Work out the finished part from the listing and answer in its coordinate system (mm). Face numbers are marked on the shaded views. A direction names the side the tool comes from. Give positions to 0.01 mm unless a question says otherwise; leave off trailing zeros. Loops run counter-clockwise (first coordinate to the right, second up) from the corner with the lowest first, then second, coordinate; pieces in that order, holes last. Notation, with made-up numbers: M -33.5,-7 L -8.5,-7 A22 ccw -8.5,28 Z; hole C 18.5,-1 d6. An arc over 180 degrees is marked long. Write item = value, one per line. Start each with the question number.
1. Flat-ended cylindrical pins translate along their axes: pin 1 Ø2 at (x, z) = (1.5, 4) entering from -Y; pin 2 Ø4.5 at (x, z) = (-14.5, 2.5) entering from +Y; pin 3 Ø3 at (y, z) = (5, 1.5) entering from +X. Find the tip coordinate at first contact, or state that the pin passes through.
2. The mould has two halves that part along X. Classify the marked faces 4, 5 and 6: released by +X, released by -X, zero draft, split by the parting line, or undercut.
3. Section B-B on z = 6.75 is taken. Determine the outline of the cut face in (x, y), plus the area to 3 significant figures.
4. Section D-D on z = 4.5 is taken. Determine the outline of the cut face in (x, y).
5. Consider L1, parallel to Y at x = 4.5, z = 7.5; L2, parallel to Z at x = -14, y = -4.7; L3, parallel to X at y = 2.5, z = 2.75. Determine where each line is inside the solid, lowest interval first. Write a range as [from, to].
6. For the marked faces 1, 2 and 3, determine the directions among +Z, -Z, +X, -X, +Y, -Y from which every point of the face is accessible in a straight line to the end or side of a thin tool.
7. Section C-C on y = -1.35 is taken. Determine the outline of the cut face in (x, z).
8. Section A-A on x = 0 is taken. Determine the outline of the cut face in (y, z), plus the area to 3 significant figures.
```python
from build123d import *

# Parameters (mm, degrees)
SKETCH3_W                                            = 18
SKETCH3_H                                            = 13
BOSS_EXTRUDE1_DEPTH                                  = 9
SKETCH9_W                                            = 12.6
SKETCH9_H                                            = 10.3
CUT_EXTRUDE2_DEPTH                                   = 6
SKETCH10_R                                           = 2.25
CUT_EXTRUDE3_DEPTH                                   = 13.619429464
CSK_FOR_M1_6_COUNTERSUNK_FLAT_HEAD_SCREW_D           = 2
CSK_FOR_M1_6_COUNTERSUNK_FLAT_HEAD_SCREW_CSINK_D     = 3.6
CSK_FOR_M1_6_COUNTERSUNK_FLAT_HEAD_SCREW_CSINK_ANGLE = 90
SKETCH14_W                                           = 9
SKETCH14_H                                           = 4
BOSS_EXTRUDE2_DEPTH                                  = 10
M1_6_CLEARANCE_HOLE1_D                               = 2


with BuildPart() as part:
    # Sketch3 → Boss-Extrude1 (new body)
    with BuildSketch(Plane.XY):
        Rectangle(SKETCH3_W, SKETCH3_H)
    extrude(amount=BOSS_EXTRUDE1_DEPTH)

    # Sketch9 → Cut-Extrude2 (cut)
    with BuildSketch(Plane(origin=(0, 0, 0), x_dir=(-1, 0, 0), z_dir=(0, 0, -1))):
        with Locations((0, -1.35)):
            Rectangle(SKETCH9_W, SKETCH9_H)
    extrude(amount=-CUT_EXTRUDE2_DEPTH, mode=Mode.SUBTRACT)

    # Sketch10 → Cut-Extrude3 (cut, through all)
    with BuildSketch(Plane(origin=(0, 0, 6), x_dir=(-1, 0, 0), z_dir=(0, 0, -1))):
        with Locations((0, -1.35)):
            Circle(SKETCH10_R)
    extrude(amount=-CUT_EXTRUDE3_DEPTH, mode=Mode.SUBTRACT)

    # CSK for M1.6 Countersunk Flat Head Screw2 (through all)
    with Locations(Plane.XY.offset(9)):
        with Locations((-4.5, -1.35), (4.5, -1.35)):
            CounterSinkHole(CSK_FOR_M1_6_COUNTERSUNK_FLAT_HEAD_SCREW_D / 2, CSK_FOR_M1_6_COUNTERSUNK_FLAT_HEAD_SCREW_CSINK_D / 2, counter_sink_angle=CSK_FOR_M1_6_COUNTERSUNK_FLAT_HEAD_SCREW_CSINK_ANGLE)

    # Sketch14 → Boss-Extrude2 (add)
    with BuildSketch(Plane(origin=(9, 0, 0), x_dir=(0, 0, -1), z_dir=(1, 0, 0))):
        with Locations((-4.5, -4.5)):
            Rectangle(SKETCH14_W, SKETCH14_H)
    boss_extrude2 = extrude(amount=BOSS_EXTRUDE2_DEPTH)

    # M1.6 Clearance Hole1 (through all)
    with Locations(Plane(origin=(0, -2.5, 0), x_dir=(1, 0, 0), z_dir=(0, 1, 0))):
        with Locations((14, -4.5)):
            m1_6_clearance_hole1 = Hole(M1_6_CLEARANCE_HOLE1_D / 2)

    # Mirror2: Boss-Extrude2, M1.6 Clearance Hole1 across plane
    add(boss_extrude2.mirror(Plane(origin=(0, 0, 0), x_dir=(0, 0, 1), z_dir=(1, 0, 0))))
    add(m1_6_clearance_hole1.mirror(Plane(origin=(0, 0, 0), x_dir=(0, 0, 1), z_dir=(1, 0, 0))), mode=Mode.SUBTRACT)


solid = part.part
```
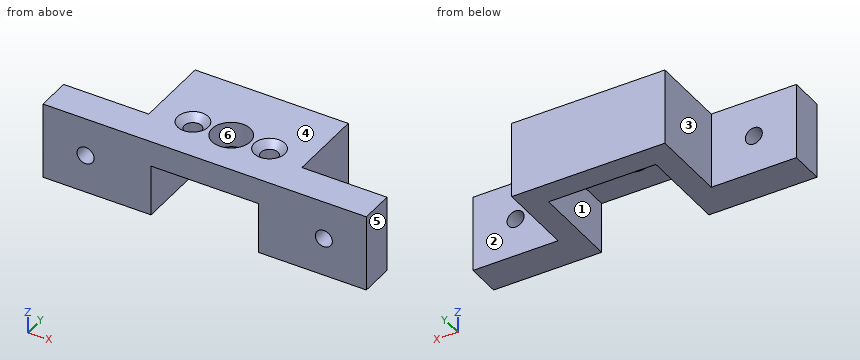
Verdict:
q1.pin_1 = 3.8
q1.pin_2 = -2.5
q1.pin_3 = 9
q2.face_4 = zero draft
q2.face_5 = released by +X
q2.face_6 = undercut
q3.outline = M -19,-6.5 L 19,-6.5 L 19,-2.5 L 9,-2.5 L 9,6.5 L -9,6.5 L -9,-2.5 L -19,-2.5 Z; hole C -4.5,-1.35 d2; hole C 0,-1.35 d4.5; hole C 4.5,-1.35 d2
q3.area = 292 mm2
q4.outline = M -19,-6.5 L -15,-6.5 L -15,-2.5 L -19,-2.5 Z; M -13,-6.5 L -6.3,-6.5 L -6.3,3.8 L 6.3,3.8 L 6.3,-6.5 L 13,-6.5 L 13,-2.5 L 9,-2.5 L 9,6.5 L -9,6.5 L -9,-2.5 L -13,-2.5 Z; M 15,-6.5 L 19,-6.5 L 19,-2.5 L 15,-2.5 Z
q5.L1 = [-6.5, -2.35], [-0.35, 6.5]
q5.L2 = [0, 3.5], [5.5, 9]
q5.L3 = [-9, -6.3], [6.3, 9]
q6.face_1 = -Z, -Y
q6.face_2 = +Z, -Z, +X, +Y
q6.face_3 = +Z, -Z, -X, +Y
q7.outline = M -9,0 L -6.3,0 L -6.3,6 L -5.5,6 L -5.5,8.2 L -6.3,9 L -9,9 Z; M -3.5,6 L -2.25,6 L -2.25,9 L -2.7,9 L -3.5,8.2 Z; M 2.25,6 L 3.5,6 L 3.5,8.2 L 2.7,9 L 2.25,9 Z; M 5.5,6 L 6.3,6 L 6.3,0 L 9,0 L 9,9 L 6.3,9 L 5.5,8.2 Z
q8.outline = M -6.5,6 L -3.6,6 L -3.6,9 L -6.5,9 Z; M 0.9,6 L 3.8,6 L 3.8,0 L 6.5,0 L 6.5,9 L 0.9,9 Z
q8.area = 41.7 mm2
